Autodesk Inventor part; units mm, degrees
ref_plane "YZ Plane" through (0, 0, 0) normal (1, 0, 0) x (0, 1, 0)
ref_plane "XZ Plane" through (0, 0, 0) normal (0, 1, 0) x (-1, 0, 0)
ref_plane "XY Plane" through (0, 0, 0) normal (0, 0, 1) x (1, 0, 0)
ref_plane "Work Plane1" through (0, 0, 0) normal (0, 0, 1) x (1, 0, 0)
ref_plane "Work Plane2" through (0, 0, 0) normal (0, 0, 1) x (1, 0, 0)
sketch "Sketch2" plane through (0, 0, 0) normal (0, 0, 1) x (1, 0, 0)
  circle A0 centre (42.5, -29.5) radius 2.15
  circle A1 centre (-37.5, -29.5) radius 2.15
  circle A2 centre (-37.5, 29.5) radius 2.15
  circle A3 centre (42.5, 29.5) radius 2.15
  line L0 (-41.5, 33.5) -> (46.5, 33.5)
  line L1 (46.5, 33.5) -> (46.5, -33.5)
  line L2 (46.5, -33.5) -> (-41.5, -33.5)
  line L3 (-41.5, -33.5) -> (-41.5, 33.5)
  line L4 (-37.5, 29.5) -> (42.5, 29.5)
  point P0 (0, 0)
  point P1 (-41.5, 0)
  point P2 (2.5, 29.5)
  point P3 (2.5, 33.5)
  dimension "d0" = 67
  dimension "d1" = 88
extrude "Extrusion1" add sketch "Sketch2" along normal blind 2
sketch "Sketch3" plane through (0, 0, 2) normal (0, 0, 1) x (1, 0, 0)
  circle A0 centre (2.5, 18.7725) radius 5
  line L0 (46.5, 33.5) -> (-41.5, 33.5)
  circle A1 centre (2.5, 27.7153) radius 3
  line L1 (-0.5, 27.7153) -> (-0.5, 22.7725)
  line L2 (5.5, 27.7153) -> (5.5, 22.7725)
  point P0 (0, 0)
  point P1 (2.5, 33.5)
  dimension "d4" = 10
  dimension "d5" = 6
extrude "Extrusion2" cut sketch "Sketch3" against normal through all
sketch "Sketch4" plane through (0, 0, 2) normal (0, 0, 1) x (1, 0, 0)
  circle A0 centre (-37.5, 29.5) radius 2.15
  circle A1 centre (-37.5, 29.5) radius 4
  line L0 (46.5, 33.5) -> (-41.5, 33.5)
  circle A2 centre (-37.5, -29.5) radius 2.15
  circle A3 centre (-37.5, -29.5) radius 4
  line L1 (-41.5, -33.5) -> (46.5, -33.5)
  circle A4 centre (42.5, -29.5) radius 2.15
  circle A5 centre (42.5, -29.5) radius 4
  circle A6 centre (42.5, 29.5) radius 2.15
  circle A7 centre (42.5, 29.5) radius 4
  point P0 (0, 0)
extrude "Extrusion3" add sketch "Sketch4" along normal blind 4
sketch "Sketch5" plane through (0, 0, 2) normal (0, 0, 1) x (1, 0, 0)
  line L0 (-41.5, -33.5) -> (46.5, -33.5)
  circle A0 centre (2.5, -33.5) radius 30
  point P0 (0, 0)
  point P1 (32.5, -33.5)
  point P2 (-27.5, -33.5)
  dimension "d10" = 60
extrude "Extrusion4" cut sketch "Sketch5" against normal through all contours A0 L0 picked at (9.9851, -22.0825)
fillet "Fillet1" radius 4 6 edges at (-41.5, 33.5, 1) (46.5, 33.5, 1) (-41.5, -33.5, 1) (46.5, -33.5, 1) (-27.5, -33.5, 1) (32.5, -33.5, 1)
properties part number "led 7 seg with sec v3 wall holder"
Work out the finished part from the listing and answer in its coordinate system (mm). A direction names the side the tool comes from. Round coordinates to 2 decimals unless told otherwise and drop trailing zeros. Loops run counter-clockwise (first coordinate to the right, second up) from the corner with the lowest first, then second, coordinate; pieces in that order, holes last. Notation, with made-up numbers: (79, 13.5) -> (99, 13.5) arc R6 ccw to (99, 19.5) -> close; hole circle Ø11 at (80.25, -17.75). An arc over 180 degrees is marked (long way). Write each question's results on one line, items separated by ' | '. Start each with the question number.
1. Given pin 1 Ø8 at (x, y) = (2.5, 18.77) entering from +Z; pin 2 Ø2 at (x, y) = (19.5, -5) entering from +Z, each flat-ended and moving along its own axis, determine where each tip first touches the part or whether it passes through.
2. Section C-C (y = 24.5) is taken. Determine the outline of the cut face in (x, z).
3. Section A-A (z = 4.75) is taken. Determine the outline of the cut face in (x, y).
4. A tool of negligible diameter and unlimited length cuts with its end or side. For faces 1 (the face through (33.64, -32.52, 0.99)), 2 (the face through (-41.5, 0, 1)), 3 (the face through (5.5, 25, 1)), 4 (the face through (-38.021, -33.466, 3.972)), from which of +Z, -Z, +X, -X, +Y, -Y can it reach the whole face along a straight path? Write none if from no direction.
5. Section B-B (x = 2.5) is taken. Determine the outline of the cut face in (y, z), plus the area to 3 significant figures.
6. For a pull along X with two mould halves and no side action, classify faces 5 (the face through (44.2, -31.2, 6)), 6 (the face through (2.566, 30.715, 1.014)), 7 (the face through (41.979, 25.534, 3.972)), 8 (the face through (-40.359, -32.297, 1.014)) as +X half, -X half, draft (parallel to the pull), parting line (faces both ways), or undercut.
7. Section D-D (x = 27) is taken. Determine the outline of the cut face in (y, z), plus the area to 3 significant figures.
8. Find the intervals of material crossed by probe 1 along Y at (x, z) = (42.5, 3.35); probe 2 along Y at (x, z) = (-37.5, 1.8); probe 3 along Z at (x, y) = (40, -12), in increasing order. Write a range as from..to.
Evaluation:
1) pin 1: passes through | pin 2: stops at z = 2
2) outline: (-41.5, 0) -> (-0.5, 0) -> (-0.5, 2) -> (-41.5, 2) -> close; (5.5, 0) -> (46.5, 0) -> (46.5, 2) -> (5.5, 2) -> close
3) outline: circle Ø8 at (-37.5, -29.5); circle Ø8 at (-37.5, 29.5); circle Ø8 at (42.5, -29.5); circle Ø8 at (42.5, 29.5); hole circle Ø4.3 at (-37.5, -29.5); hole circle Ø4.3 at (-37.5, 29.5); hole circle Ø4.3 at (42.5, -29.5); hole circle Ø4.3 at (42.5, 29.5)
4) face 1: +Z, -Z, -Y | face 2: +Z, -Z, -X, +Y, -Y | face 3: +Z, -Z | face 4: +Z
5) outline: (-3.5, 0) -> (13.77, 0) -> (13.77, 2) -> (-3.5, 2) -> close; (30.72, 0) -> (33.5, 0) -> (33.5, 2) -> (30.72, 2) -> close | area: 40.1 mm2
6) face 5: draft | face 6: undercut | face 7: undercut | face 8: -X half
7) outline: (-16.19, 0) -> (33.5, 0) -> (33.5, 2) -> (-16.19, 2) -> close | area: 99.4 mm2
8) probe 1: y = -33.5..-31.65, -27.35..-25.5, 25.5..27.35, 31.65..33.5 | probe 2: y = -33.5..-31.65, -27.35..27.35, 31.65..33.5 | probe 3: z = 0..2
